```python
from build123d import *

# Parameters (mm, degrees)
SKIZZE1_W                            = 57
SKIZZE1_H                            = 123
AUFSATZ_LINEAR_AUSTRAGEN1_DEPTH      = 2.5
SCHNITT_LINEAR_AUSTRAGEN1_DEPTH      = 84.889808678
SCHNITT_LINEAR_AUSTRAGEN2_DEPTH      = 68.828828679
SCHNITT_LINEAR_AUSTRAGEN3_DEPTH      = 70.726045338
SCHNITT_LINEAR_AUSTRAGEN3_DEPTH_BACK = 70.726045338
SCHNITT_LINEAR_AUSTRAGEN4_DEPTH      = 70.47454308
SCHNITT_LINEAR_AUSTRAGEN4_DEPTH_BACK = 70.47454308
SKIZZE9_W                            = 45.241474544
SKIZZE9_H                            = 11.280630507
AUFSATZ_LINEAR_AUSTRAGEN2_DEPTH      = 13
SCHNITT_LINEAR_AUSTRAGEN5_DEPTH      = 20
SKIZZE12_W                           = 36.023643564
SKIZZE12_H                           = 10.472363364
AUFSATZ_LINEAR_AUSTRAGEN3_DEPTH      = 5
SCHNITT_LINEAR_AUSTRAGEN6_DEPTH      = 12
SCHNITT_LINEAR_AUSTRAGEN8_DEPTH      = 0.5
SCHNITT_LINEAR_AUSTRAGEN8_DEPTH_BACK = 1.65
SKIZZE16_R                           = 3.1
SCHNITT_LINEAR_AUSTRAGEN9_DEPTH      = 1.15
SCHNITT_LINEAR_AUSTRAGEN9_DEPTH_BACK = 1
SKIZZE17_R                           = 3.1
SCHNITT_LINEAR_AUSTRAGEN10_DEPTH     = 10


with BuildPart() as part:
    # Skizze1 → Aufsatz-Linear austragen1 (new body)
    with BuildSketch(Plane(origin=(0, 0, 0), x_dir=(1, 0, 0), z_dir=(0, 1, 0))):
        Rectangle(SKIZZE1_W, SKIZZE1_H)
    extrude(amount=AUFSATZ_LINEAR_AUSTRAGEN1_DEPTH)

    # Skizze2 → Schnitt-Linear austragen1 (cut, through all)
    with BuildSketch(Plane(origin=(28.5, 0, 0), x_dir=(0, 0, -1), z_dir=(1, 0, 0))):
        Polygon((-61.5, 2.5), (-61.5, 0), (-60.968608596, 0), align=None)
    extrude(amount=-SCHNITT_LINEAR_AUSTRAGEN1_DEPTH, mode=Mode.SUBTRACT)

    # Skizze3 → Schnitt-Linear austragen2 (cut, through all)
    with BuildSketch(Plane(origin=(0, 2.5, 0), x_dir=(1, 0, 0), z_dir=(0, 1, 0))):
        Polygon((-28.5, -61.5), (-17.738894386, 61.5), (-28.5, 61.5), align=None)
        Polygon((28.5, -61.5), (17.738894386, 61.5), (28.5, 61.5), align=None)
    extrude(amount=-SCHNITT_LINEAR_AUSTRAGEN2_DEPTH, mode=Mode.SUBTRACT)

    # Skizze5 → Schnitt-Linear austragen3 (cut, two sides: drawn at the far end of the back side and taken through both)
    with BuildSketch(Plane(origin=(0.175618176, 0, 2.007324937), x_dir=(0, -1, 0), z_dir=(0.08715574274765484, 0, 0.9961946980917459)).offset(-SCHNITT_LINEAR_AUSTRAGEN3_DEPTH_BACK)):
        Polygon((0.008562414, 23.031470717), (-2.5, 23.031470717), (0, 21.995936811), align=None)
    extrude(amount=SCHNITT_LINEAR_AUSTRAGEN3_DEPTH + SCHNITT_LINEAR_AUSTRAGEN3_DEPTH_BACK, mode=Mode.SUBTRACT)

    # Skizze6 → Schnitt-Linear austragen4 (cut, two sides: drawn at the far end of the back side and taken through both)
    with BuildSketch(Plane(origin=(-0.152372814, 0, 1.741629235), x_dir=(0, 1, 0), z_dir=(-0.08715574274766175, 0, 0.9961946980917452)).offset(-SCHNITT_LINEAR_AUSTRAGEN4_DEPTH_BACK)):
        Polygon((2.5, 23.031470717), (0, 21.995936811), (0, 23.031470717), align=None)
    extrude(amount=SCHNITT_LINEAR_AUSTRAGEN4_DEPTH + SCHNITT_LINEAR_AUSTRAGEN4_DEPTH_BACK, mode=Mode.SUBTRACT)

    # Skizze9 → Aufsatz-Linear austragen2 (add)
    with BuildSketch(Plane.XZ):
        with Locations((0, 52.468608596)):
            Rectangle(SKIZZE9_W, SKIZZE9_H)
    extrude(amount=AUFSATZ_LINEAR_AUSTRAGEN2_DEPTH)

    # Skizze11 → Schnitt-Linear austragen5 (cut)
    with BuildSketch(Plane(origin=(0, 0, 46.828293342), x_dir=(-1, 0, 0), z_dir=(0, 0, -1))):
        Polygon((-22.620737272, -9.484039906), (0, 0), (22.620737272, -9.484039906), (22.620737272, -13), (-22.620737272, -13), align=None)
    extrude(amount=-SCHNITT_LINEAR_AUSTRAGEN5_DEPTH, mode=Mode.SUBTRACT)

    # Skizze12 → Aufsatz-Linear austragen3 (add)
    with BuildSketch(Plane.XZ):
        with Locations((0, -20.5)):
            Rectangle(SKIZZE12_W, SKIZZE12_H)
    extrude(amount=AUFSATZ_LINEAR_AUSTRAGEN3_DEPTH)

    # Skizze13 → Schnitt-Linear austragen6 (cut)
    with BuildSketch(Plane(origin=(0, 0, -25.736181682), x_dir=(-1, 0, 0), z_dir=(0, 0, -1))):
        Polygon((-18.011821782, -2.5), (-7.183132097, 0), (7.183132097, 0), (18.011821782, -2.5), (18.011821782, -5), (-18.011821782, -5), align=None)
    extrude(amount=-SCHNITT_LINEAR_AUSTRAGEN6_DEPTH, mode=Mode.SUBTRACT)

    # Skizze16 → Schnitt-Linear austragen8 (cut, two sides: drawn at the far end of the back side and taken through both)
    with BuildSketch(Plane.XZ.offset(-SCHNITT_LINEAR_AUSTRAGEN8_DEPTH_BACK)):
        with Locations(Location((12.59747694, -20.5, 0), (0, 0, 270))):
            Circle(SKIZZE16_R)
        with Locations(Location((-12.59747694, -20.5, 0), (0, 0, 270))):
            Circle(SKIZZE16_R)
    extrude(amount=SCHNITT_LINEAR_AUSTRAGEN8_DEPTH + SCHNITT_LINEAR_AUSTRAGEN8_DEPTH_BACK, mode=Mode.SUBTRACT)

    # Skizze17 → Schnitt-Linear austragen9 (cut, two sides: drawn at the far end of the back side and taken through both)
    with BuildSketch(Plane(origin=(0, -4.742019953, 0), x_dir=(1, 0, 0), z_dir=(0, 1, 0)).offset(-SCHNITT_LINEAR_AUSTRAGEN9_DEPTH_BACK)):
        with Locations(Location((-16.965552954, -52.468608596, 0), (0, 0, 270))):
            Circle(SKIZZE17_R)
        with Locations(Location((16.965552954, -52.468608596, 0), (0, 0, 270))):
            Circle(SKIZZE17_R)
    extrude(amount=SCHNITT_LINEAR_AUSTRAGEN9_DEPTH + SCHNITT_LINEAR_AUSTRAGEN9_DEPTH_BACK, mode=Mode.SUBTRACT)

    # Skizze18 → Schnitt-Linear austragen10 (cut)
    with BuildSketch(Plane(origin=(0, 2.5, 0), x_dir=(1, 0, 0), z_dir=(0, 1, 0))):
        with BuildLine():
            Line((17.738894386, 61.5), (9.738894386, 61.5))
            Line((9.738894386, 61.5), (9.738894386, 42.5))
            Line((9.738894386, 42.5), (9.738894386, 42.494341137))
            ThreePointArc((9.738894386, 42.494341137), (12.722062254, 35.369450483), (19.891707751, 32.495508801))
            Line((19.891707751, 32.495508801), (20.275944794, 32.501381142))
            Line((20.275944794, 32.501381142), (17.738894386, 61.5))
        make_face()
    extrude(amount=-SCHNITT_LINEAR_AUSTRAGEN10_DEPTH, mode=Mode.SUBTRACT)


solid = part.part
```
Input: part model. Units: mm. Frame: model coordinates. A direction names the side the tool comes from. Give positions to 0.01 mm unless a question says otherwise; leave off trailing zeros. Loops run counter-clockwise (first coordinate to the right, second up) from the corner with the lowest first, then second, coordinate; pieces in that order, holes last. Notation, with made-up numbers: (-8.5, 43) -> (5.5, 43) arc R12 ccw to (5.5, 54) -> close; hole circle Ø10 at (-20, -10.5). An arc over 180 degrees is marked (long way). Use a Markdown table: item, result.
Q1. Access query for faces 5 (the flat face through (-12.522, -1.232, -20.573)), 6 (the flat face through (-18.012, -1, -21)), 7 (the flat face through (-11.152, -4.676, 52.39)), 8 (the flat face through (15, -1, -15.264)), 9 (the flat face through (-22.621, -5, 52)). Directions: +Z, -Z, +X, -X, +Y, -Y. A direction counts if a zero-diameter tool reaches every point of the face in a straight line with its end or side. Return the directions, or none.
Entries:
| item | result |
|---|---|
| face 5 | -Z, -Y |
| face 6 | -Z, -X, -Y |
| face 7 | +Z, -Z, -Y |
| face 8 | +X, -X, -Y |
| face 9 | +Z, -Z, -X, -Y |
Q2. Pull-direction query (Z, two-part tool) for faces 1 (the flat face through (18.012, -1, -21)), 2 (the flat face through (-14, -1, -25.736)), 3 (the flat face through (13, -0.5, -20)), 4 (the flat face through (-14, -4, 58.109)); classes: pulls with the +Z half, pulls with the -Z half, needs draft (parallel to the pull), parting line crosses it, or undercut.
Entries:
| item | result |
|---|---|
| face 1 | needs draft |
| face 2 | pulls with the -Z half |
| face 3 | undercut |
| face 4 | pulls with the +Z half |
Q3. Ray query, probe 1 along Z at (x, y) = (-14, -0.75); probe 2 along X at (y, z) = (0.6, -20.5); probe 3 along X at (y, z) = (0.35, -20.5). Return the intervals inside material, ascending. Write a range as from..to.
Entries:
| item | result |
|---|---|
| probe 1 | z = -25.74..-15.26, 46.83..58.11 |
| probe 2 | x = -20.54..-15.7, -9.5..9.5, 15.7..20.54 |
| probe 3 | x = -20.43..-15.7, -9.5..9.5, 15.7..20.43 |
Q4. Section query A-A, the plane z = -20.5. Return the cut outline in (x, y), plus the area to 3 significant figures.
Entries:
| item | result |
|---|---|
| outline | (-21.33, 2.5) -> (-20.29, 0) -> (-18.01, 0) -> (-18.01, -2.5) -> (-7.18, 0) -> (7.18, 0) -> (18.01, -2.5) -> (18.01, 0) -> (20.29, 0) -> (21.33, 2.5) -> close; hole (-15.7, -0.5) -> (-9.5, -0.5) -> (-9.5, 1.65) -> (-15.7, 1.65) -> close; hole (9.5, -0.5) -> (15.7, -0.5) -> (15.7, 1.65) -> (9.5, 1.65) -> close |
| area | 104 mm² |
Q5. First-contact query: P1, Ø0.8, axis at y = -1, z = -20, coming from the +X side; P2, Ø3, axis at x = 12.5, y = -1, coming from the +Z side; P3, Ø10, axis at x = -16.97, z = 52.47, coming from the -Y side. Flat tips, straight axial feed; report the tip coordinate or a pass-through.
Entries:
| item | result |
|---|---|
| P1 | stops at x = 18.01 |
| P2 | stops at z = 61.07 |
| P3 | stops at y = -9.21 |
Q6. Section query B-B, the plane z = -34.5. Return the cut outline in (x, y).
Entries:
| item | result |
|---|---|
| outline | (-20.1, 2.5) -> (-19.06, 0) -> (13.73, 0) -> (13.73, 2.5) -> close |
